from build123d import *

# Parameters (mm, degrees)
F1_DEPTH = 25.4
F3_DEPTH = 25.4


with BuildPart() as f1:
    # F0 (on Front) → F1 (new body)
    with BuildSketch(Plane.XZ):
        Polygon((-58.37366, 14.244376), (0, 0), (-16.961619, 49.44808), align=None)
    extrude(amount=F1_DEPTH)

    # F2 (on face) → F3 (join)
    with BuildSketch(Plane.XZ.offset(25.4)):
        Polygon((8.147058, 28.529268), (-65.254316, 41.173346), (-58.37366, 14.244376), (0, 0), align=None)
    extrude(amount=-F3_DEPTH)


solid = f1.part
Here's how the part is built. I have some questions about the finished solid (model axes, mm). A direction names the side the tool comes from. Coordinates: 2 decimals unless noted, no trailing zeros. Write each loop counter-clockwise with the first axis right and the second up, starting at its lowest first coordinate (ties: lowest second). Pieces come first, ordered by that corner, then holes.
Item 1: If I drill on line 1 (Z direction, x = -26.5, y = -11.5); line 2 (X direction, y = -15.75, z = 21); line 3 (Z direction, x = -57.5, y = -3.25), over which ranges is the centre line in solid material (lowest first)?
Item 2: On a 3-axis mill with a long thin cutter (end or side, diameter ignored), from which of +Z, -Z, +X, -X, +Y, -Y can I reach the whole of each face in a straight line? I mean faces 1 (the flat face through (-29, 0, 25)), 2 (the flat face through (-48.999, -12.878, 38.373)). Say none if no direction works.
Item 3: I want a section at A-A on z = 39. Write out the boundary of the cut face in (x, y).
Item 4: Will these pins go through, and if not, where does the flat tip stop? pin 1 (6 mm diameter, centred on x = -19, z = 41, fed in from +Y); pin 2 (1.5 mm diameter, centred on x = -26, y = -8, fed in from -Z); pin 3 (2 mm diameter, centred on x = -9, y = -15, fed in from -Z); pin 4 (2 mm diameter, centred on x = -19, y = -12, fed in from -Z).
Item 5: If we mould it in two halves opening along X, with no side actions, what happens to faces 3 (the flat face through (4, -13, 14)), 4 (the flat face through (-24.96, -12.52, 42.65)), 5 (the flat face through (-29, -25.4, 25))? For each: +X half, -X half, draft (parallel to the pull), parting line (faces both ways), or undercut.
Item 6: I want a section at D-D on z = 22. Write out the boundary of the cut face in (x, y).
Item 7: I want a section at B-B on y = -15.25. Write out the boundary of the cut face in (x, z).
Item 8: I want a section at C-C on x = -50. Write out the boundary of the cut face in (y, z), and give its area (3 significant figures).
Findings below:
1. line 1: z = 6.47 to 41.34
1. line 2: x = -60.1 to 6
1. line 3: z = 14.03 to 39.84
2. face 1: +Z, -Z, +X, -X, +Y
2. face 2: +Z, +Y, -Y
3. outline: (-64.7, -25.4) - (-52.64, -25.4) - (-52.64, 0) - (-64.7, 0) - close; (-29.25, -25.4) - (-13.38, -25.4) - (-13.38, 0) - (-29.25, 0) - close
4. pin 1: stops at y = 0
4. pin 2: stops at z = 6.16
4. pin 3: stops at z = 1.95
4. pin 4: stops at z = 4.39
5. face 3: +X half
5. face 4: undercut
5. face 5: draft
6. outline: (-60.36, -25.4) - (6.28, -25.4) - (6.28, 0) - (-60.36, 0) - close
7. outline: (-65.25, 41.17) - (-58.37, 14.24) - (0, 0) - (8.15, 28.53) - (-10.91, 31.81) - (-16.96, 49.45) - (-33.19, 35.65) - close
8. outline: (-25.4, 12.2) - (0, 12.2) - (0, 38.55) - (-25.4, 38.55) - close
8. area: 669 mm2
